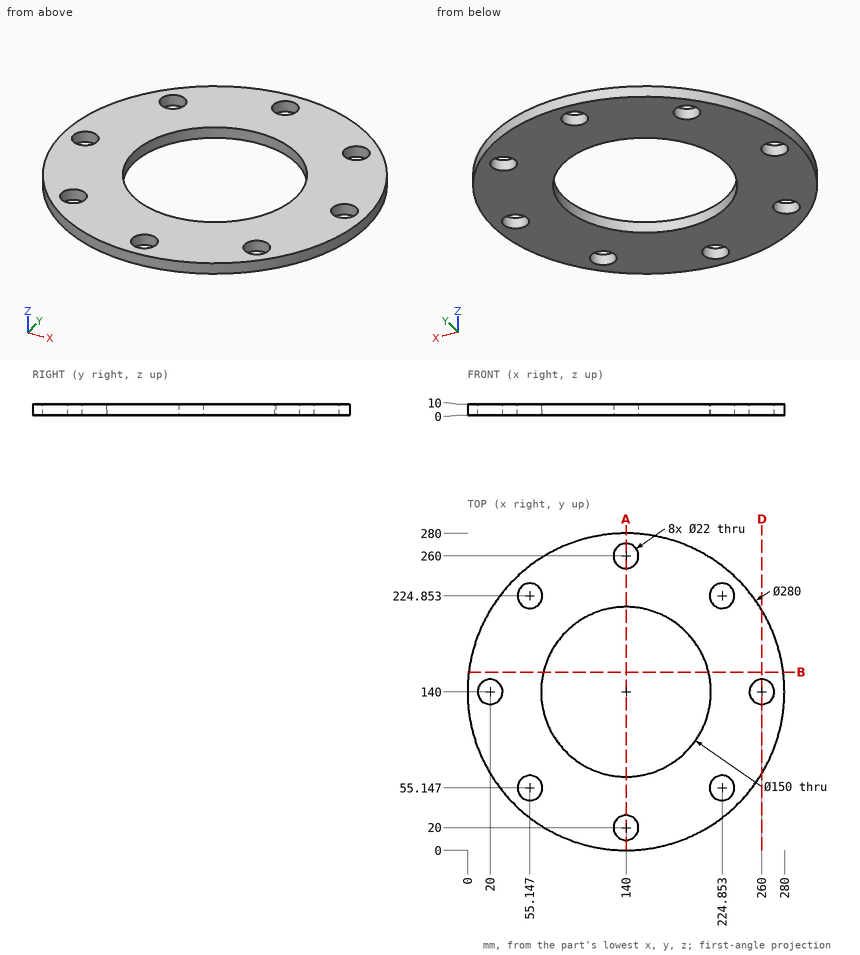
Geometry check sheet. Reference: drawing and pictorial views, mm from the part's lowest x, y, z. Round coordinates to 2 decimals unless told otherwise and drop trailing zeros. Order: outer loops, then holes, each group sorted by start corner. A loop starts at its lowest first (then second) coordinate and runs counter-clockwise, first axis right, second up.
Q1. Cross-section at A-A, the plane x = 140. Enter the section's corners in (y, z).
Filled sheet:
outline: (0, 0) - (9, 0) - (9, 10) - (0, 10) - close; (31, 0) - (65, 0) - (65, 10) - (31, 10) - close; (215, 0) - (249, 0) - (249, 10) - (215, 10) - close; (271, 0) - (280, 0) - (280, 10) - (271, 10) - close
Q2. Cross-section at D-D, the plane x = 260. Enter the section's corners in (y, z), plus the area to 3 significant figures.
Filled sheet:
outline: (67.89, 0) - (129, 0) - (129, 10) - (67.89, 10) - close; (151, 0) - (212.11, 0) - (212.11, 10) - (151, 10) - close
area: 1,220 mm2
Q3. Scan lines: L1, parallel to Y at x = 140, z = 4; L2, parallel to X at y = 61.5, z = 6.75; L3, parallel to Y at x = 216, z = 5.75 (1 decimal). Record each from-to range of solid material in increasing order.
Filled sheet:
L1: y = 0 to 9, 31 to 65, 215 to 249, 271 to 280
L2: x = 24.08 to 46.17, 64.13 to 215.87, 233.83 to 255.92
L3: y = 22.4 to 48.6, 61.7 to 218.3, 231.4 to 257.6
Q4. Depth check by flat-ended pin: P1, Ø13, axis at x = 140, y = 260, coming from the +Z side; P2, Ø3, axis at x = 43, z = 8, coming from the +Y side; P3, Ø4, axis at x = 82.5, z = 9, coming from the -Y side. Enter the tip coordinate at first touch or a pass-through.
Filled sheet:
P1: passes through
P2: stops at y = 242.37
P3: stops at y = 11.47
Q5. Cross-section at B-B, the plane y = 157.5. Enter the section's corners in (x, z).
Filled sheet:
outline: (1.1, 0) - (67.07, 0) - (67.07, 10) - (1.1, 10) - close; (212.93, 0) - (278.9, 0) - (278.9, 10) - (212.93, 10) - close
